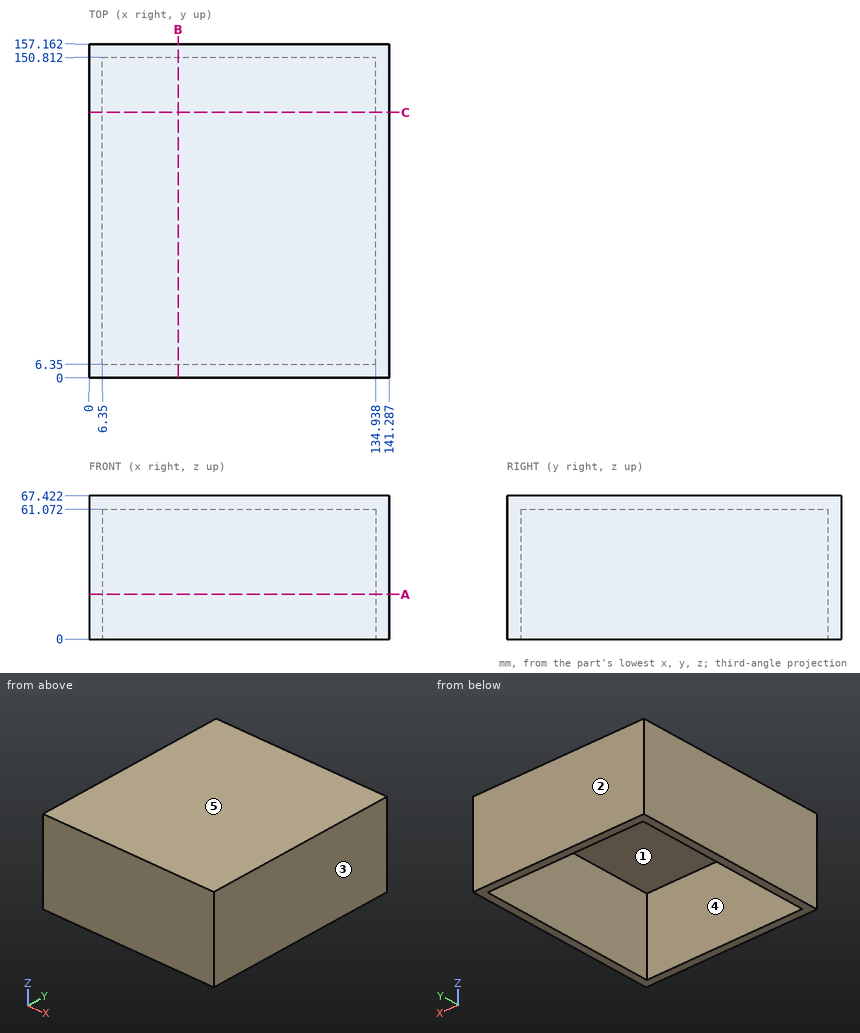
The figure shows three views and two pictorial views of one solid part (mm, origin at its lowest corner). Answer the questions. A direction names the side the tool comes from. Coordinates: 2 decimals unless noted, no trailing zeros. Order: outer loops, then holes, each group sorted by start corner. A loop starts at its lowest first (then second) coordinate and runs counter-clockwise, first axis right, second up.
Q1. Consider line 1 (Y direction, x = 49, z = 46.5); line 2 (X direction, y = 46, z = 8.5); line 3 (Z direction, x = 52, y = 9.5). Determine where each line is inside the solid, lowest interval first.
Q2. A cutting plane is placed at A-A, the plane z = 21. Write down the section's boundary in (x, y), and give its area (3 significant figures).
Q3. Which of the six approach directions +Z, -Z, +X, -X, +Y, -Y give full straight-line access (tool end or side, diameter ignored) to the marked faces 4 and 5?
Q4. For a pull along X with two mould halves and no side action, classify the marked faces 1, 2 and 3 as pulls with the +X half, pulls with the -X half, needs draft (parallel to the pull), parting line crosses it, or undercut.
Q5. Given P1, Ø8, axis at x = 99, y = 83.5, coming from the -Z side, flat-ended and moving along its own axis, determine where the tip first touches the part or whether it passes through.
Q6. A cutting plane is placed at C-C, the plane y = 125. Write down the section's boundary in (x, z), and give its area (3 significant figures).
Q7. A cutting plane is placed at B-B, the plane x = 42. Write down the section's boundary in (y, z).
Answers follow:
1. line 1: y = 0 to 6.35, 150.81 to 157.16
1. line 2: x = 0 to 6.35, 134.94 to 141.29
1. line 3: z = 61.07 to 67.42
2. outline: (0, 0) - (141.29, 0) - (141.29, 157.16) - (0, 157.16) - close; hole (6.35, 6.35) - (134.94, 6.35) - (134.94, 150.81) - (6.35, 150.81) - close
2. area: 3,630 mm2
3. face 4: -Z
3. face 5: +Z, +X, -X, +Y, -Y
4. face 1: undercut
4. face 2: needs draft
4. face 3: pulls with the +X half
5. P1: stops at z = 61.07
6. outline: (0, 0) - (6.35, 0) - (6.35, 61.07) - (134.94, 61.07) - (134.94, 0) - (141.29, 0) - (141.29, 67.42) - (0, 67.42) - close
6. area: 1,670 mm2
7. outline: (0, 0) - (6.35, 0) - (6.35, 61.07) - (150.81, 61.07) - (150.81, 0) - (157.16, 0) - (157.16, 67.42) - (0, 67.42) - close
